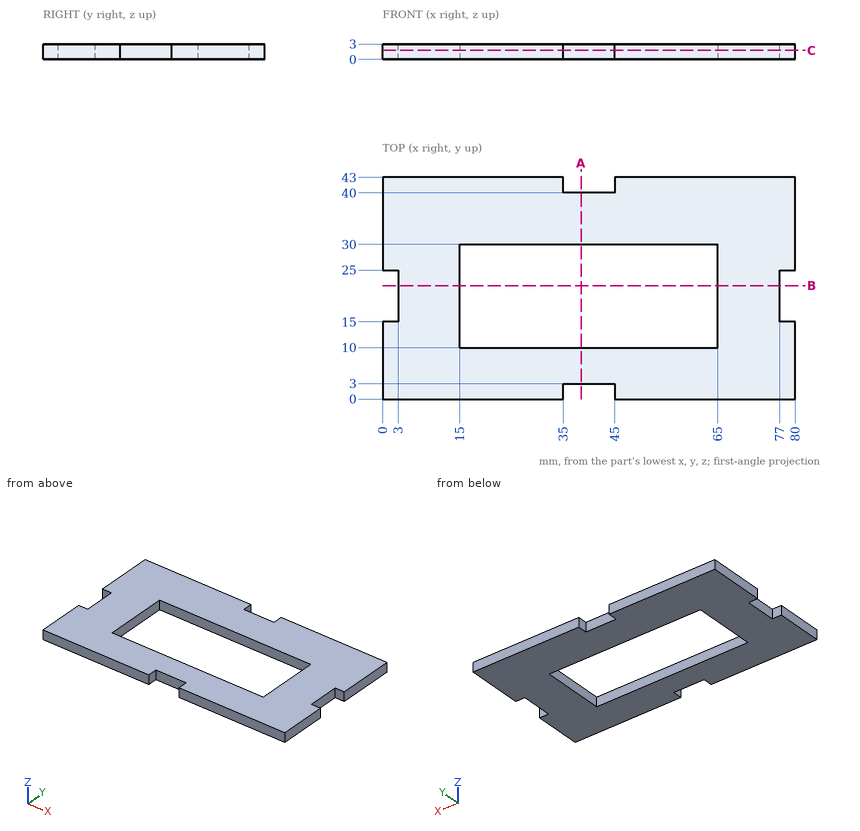
Print and shaded views of the part. All mm, measured from the part's lowest x, y and z. Give positions to 0.01 mm unless a question says otherwise; leave off trailing zeros. Loops run counter-clockwise (first coordinate to the right, second up) from the corner with the lowest first, then second, coordinate; pieces in that order, holes last.
1) Saw through at A-A (x = 38.5). Write the cut outline in (y, z), plus the area to 3 significant figures.
2) Wall check: line 1 (Y direction, x = 40, z = 2.05); line 2 (Y direction, x = 20.5, z = 2.35); line 3 (X direction, y = 22.5, z = 2.2). Give the ranges that are in metal, low to high.
3) Saw through at C-C (z = 1.75). Write the cut outline in (x, y).
4) Saw through at B-B (y = 22). Write the cut outline in (x, z).
5) Flat gauge pins, fed straight in: pin 1 Ø12 at (x, y) = (18.5, 12) entering from -Z; pin 2 Ø1 at (x, z) = (40.5, 1) entering from +Y; pin 3 Ø0.9 at (y, z) = (20.5, 2) entering from -X; pin 4 Ø0.9 at (x, z) = (41, 2) entering from -Y. Where does each tip first touch, or does it go through?
Answer block:
1. outline: (3, 0) - (10, 0) - (10, 3) - (3, 3) - close; (30, 0) - (40, 0) - (40, 3) - (30, 3) - close
1. area: 51.0 mm2
2. line 1: y = 3 to 10, 30 to 40
2. line 2: y = 0 to 10, 30 to 43
2. line 3: x = 3 to 15, 65 to 77
3. outline: (0, 0) - (35, 0) - (35, 3) - (45, 3) - (45, 0) - (80, 0) - (80, 15) - (77, 15) - (77, 25) - (80, 25) - (80, 43) - (45, 43) - (45, 40) - (35, 40) - (35, 43) - (0, 43) - (0, 25) - (3, 25) - (3, 15) - (0, 15) - close; hole (15, 10) - (65, 10) - (65, 30) - (15, 30) - close
4. outline: (3, 0) - (15, 0) - (15, 3) - (3, 3) - close; (65, 0) - (77, 0) - (77, 3) - (65, 3) - close
5. pin 1: stops at z = 0
5. pin 2: stops at y = 40
5. pin 3: stops at x = 3
5. pin 4: stops at y = 3
